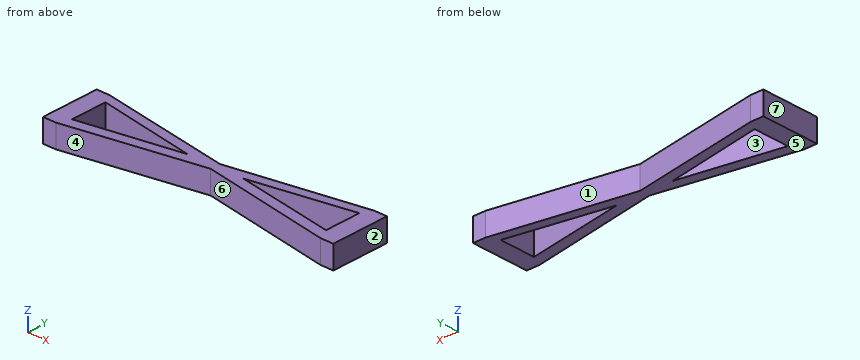
from build123d import *

# Parameters (mm, degrees)
BOSS_EXTRUDE1_DEPTH = 19.0272625


with BuildPart() as part:
    # Sketch1 → Boss-Extrude1 (new body)
    with BuildSketch(Plane.XY):
        Polygon((0, 0), (10.985406775, 0), (123.4989795, 20.769522906), (236.012552225, 0), (246.997959, 0), (246.997959, 49.45), (236.267497729, 49.45), (123.4989795, 29.326227234), (10.730461271, 49.45), (0, 49.45), align=None)
        Polygon((15.5, 40.705671267), (99.929892015, 25.120275357), (15.5, 10.053588411), align=None, mode=Mode.SUBTRACT)
        Polygon((231.497959, 40.705671267), (147.068066985, 25.120275357), (231.497959, 10.053588411), align=None, mode=Mode.SUBTRACT)
    extrude(amount=BOSS_EXTRUDE1_DEPTH)


solid = part.part
Verification items for the finished model (mm, model axes). Face numbers are marked on the shaded views. A direction names the side the tool comes from. Give positions to 0.01 mm unless a question says otherwise; leave off trailing zeros. Write each loop counter-clockwise with the first axis right and the second up, starting at its lowest first coordinate (ties: lowest second). Pieces come first, ordered by that corner, then holes. Notation, with made-up numbers: (80.5, 62.25) - (137.5, 62.25) arc R19 cw to (137.5, 99.25) - close; hole circle Ø5 at (-23, 12.25). An arc over 180 degrees is marked (long way). Answer as CSV lines item,"result". Start each with the question number.
1. Sectioned sample at B-B (x = 29). Record the boundary of the cut face in (y, z), then the cut area to 3 significant figures.
2. Sectioned sample at C-C (z = 5.5). Record the boundary of the cut face in (x, y), then the cut area to 3 significant figures.
3. Draft check along X on the marked faces 5, 6 and 7. Enter one of: pulls with the +X half, pulls with the -X half, needs draft (parallel to the pull), parting line crosses it, or undercut.
4. Thickness scan on line 1 (Y direction, x = 68, z = 9.75); line 2 (Y direction, x = 147.5, z = 16.5); line 3 (Y direction, x = 125.5, z = 1). Record the ranges inside material, lowest first.
5. Sectioned sample at A-A (y = 6). Record the boundary of the cut face in (x, z), then the cut area to 3 significant figures.
6. Sectioned sample at D-D (y = 36.5). Record the boundary of the cut face in (x, z), then the cut area to 3 significant figures.
7. Depth check by flat-ended pin: pin 1 (1 mm diameter, centred on x = 87, z = 9, fed in from +Y); pin 2 (6 mm diameter, centred on x = 164.5, z = 13, fed in from +Y); pin 3 (2 mm diameter, centred on x = 105, y = 16, fed in from +Z); pin 4 (3 mm diameter, centred on x = 128.5, z = 6.5, fed in from +Y). Enter the tip coordinate at first touch or a pass-through.
8. Set-up check for the marked faces 1, 2, 3 and 4: record each of +Z, -Z, +X, -X, +Y, -Y from which the full face is reachable in a straight line by a thin tool's end or side.
Derived:
1,outline,"(3.33, 0) - (12.46, 0) - (12.46, 19.03) - (3.33, 19.03) - close; (38.21, 0) - (46.19, 0) - (46.19, 19.03) - (38.21, 19.03) - close"
1,area,"326 mm²"
2,outline,"(0, 0) - (10.99, 0) - (123.5, 20.77) - (236.01, 0) - (247, 0) - (247, 49.45) - (236.27, 49.45) - (123.5, 29.33) - (10.73, 49.45) - (0, 49.45) - close; hole (15.5, 10.05) - (99.93, 25.12) - (15.5, 40.71) - close; hole (147.07, 25.12) - (231.5, 10.05) - (231.5, 40.71) - close"
2,area,"5,020 mm²"
3,face 5,"needs draft"
3,face 6,"undercut"
3,face 7,"pulls with the -X half"
4,line 1,"10.52 to 19.42, 31.01 to 39.23"
4,line 2,"16.34 to 25.04, 25.2 to 33.61"
4,line 3,"20.4 to 29.68"
5,outline,"(0, 0) - (43.49, 0) - (43.49, 19.03) - (0, 19.03) - close; (203.51, 0) - (247, 0) - (247, 19.03) - (203.51, 19.03) - close"
5,area,"1,650 mm²"
6,outline,"(0, 0) - (15.5, 0) - (15.5, 19.03) - (0, 19.03) - close; (38.28, 0) - (83.3, 0) - (83.3, 19.03) - (38.28, 19.03) - close; (163.7, 0) - (208.71, 0) - (208.71, 19.03) - (163.7, 19.03) - close; (231.5, 0) - (247, 0) - (247, 19.03) - (231.5, 19.03) - close"
6,area,"2,300 mm²"
7,pin 1,"y = 35.93"
7,pin 2,"y = 37.18"
7,pin 3,"through"
7,pin 4,"y = 30.49"
8,face 1,"+Z, -Z, +Y"
8,face 2,"+Z, -Z, +X, +Y, -Y"
8,face 3,"+Z, -Z"
8,face 4,"+Z, -Z, -Y"
